Read the model definition and answer for the solid it produces. Units are mm, in the model's axes. A direction names the side the tool comes from. Give positions to 0.01 mm unless a question says otherwise; leave off trailing zeros. Write each loop counter-clockwise with the first axis right and the second up, starting at its lowest first coordinate (ties: lowest second). Pieces come first, ordered by that corner, then holes. Notation, with made-up numbers: (-29.5, -23) - (24.5, -23) arc R24 ccw to (24.5, 12) - close; hole circle Ø5 at (29, 60). An arc over 180 degrees is marked (long way). Answer as CSV lines item,"result".
```python
from build123d import *

# Parameters (mm, degrees)
F1_DEPTH      = 9
F1_DEPTH_BACK = 9
F3_DEPTH      = 25
F3_DEPTH_BACK = 25
F5_DEPTH      = 25
F5_DEPTH_BACK = 25
F6_R          = 2.5
F7_DEPTH      = 25
F7_DEPTH_BACK = 25


with BuildPart() as f1:
    # F0 (on Top) → F1 (new body, two sides)
    with BuildSketch(Plane.XY) as f1_sk:
        with BuildLine():
            ThreePointArc((-0.5590957934, 20), (-0.139801245, 10.0039065883), (0, 0))
            ThreePointArc((0, 0), (-0.139801245, -10.0039065883), (-0.5590957934, -20))
            Line((-0.5590957934, -20), (39, -20))
            Line((39, -20), (39, 20))
            Line((39, 20), (-0.5590957934, 20))
        make_face()
    extrude(amount=F1_DEPTH)
    extrude(f1_sk.sketch, amount=-F1_DEPTH_BACK)

    # F2 (on Front) → F3 (cut, two sides)
    with BuildSketch(Plane.XZ) as f3_sk:
        with BuildLine():
            Line((-2.6374068111, -9), (24, -9))
            Line((24, -9), (17.9378221735, 1.5))
            ThreePointArc((17.9378221735, 1.5), (16.1076951546, 3.3301270189), (13.6076951546, 4))
            Line((13.6076951546, 4), (-2.6374068111, 4))
            Line((-2.6374068111, 4), (-2.6374068111, -9))
        make_face()
    extrude(amount=-F3_DEPTH, mode=Mode.SUBTRACT)
    extrude(f3_sk.sketch, amount=F3_DEPTH_BACK, mode=Mode.SUBTRACT)

    # F4 (on Top) → F5 (cut, two sides)
    with BuildSketch(Plane.XY) as f5_sk:
        with BuildLine():
            ThreePointArc((19, -5), (20.4644660941, -8.5355339059), (24, -10))
            Line((24, -10), (41.5962561965, -10))
            Line((41.5962561965, -10), (41.5962561965, 10))
            Line((41.5962561965, 10), (24, 10))
            ThreePointArc((24, 10), (20.4644660941, 8.5355339059), (19, 5))
            Line((19, 5), (19, 0))
            Line((19, 0), (19, -5))
        make_face()
    extrude(amount=-F5_DEPTH, mode=Mode.SUBTRACT)
    extrude(f5_sk.sketch, amount=F5_DEPTH_BACK, mode=Mode.SUBTRACT)

    # F6 (on Front) → F7 (cut, two sides)
    with BuildSketch(Plane.XZ) as f7_sk:
        with Locations((32, -5)):
            Circle(F6_R)
    extrude(amount=-F7_DEPTH, mode=Mode.SUBTRACT)
    extrude(f7_sk.sketch, amount=F7_DEPTH_BACK, mode=Mode.SUBTRACT)


solid = f1.part
```
(1) A cutting plane is placed at B-B (x = 28). Write down the section's boundary in (y, z), and give its area (3 significant figures).
Worked out:
outline,"(-20, -9) - (-10, -9) - (-10, 9) - (-20, 9) - close; (10, -9) - (20, -9) - (20, 9) - (10, 9) - close"
area,"360 mm^2"
(2) The mould has two halves that part along X. Classify faces 4 (the flat face through (31, 15, -9)), 5 (the flat face through (18.32, -0.28, 0.84)), 6 (the cylindrical face through (31.67, -14.93, -2.52)): +X half, -X half, draft (parallel to the pull), parting line (faces both ways), or undercut.
Worked out:
face 4,"draft"
face 5,"-X half"
face 6,"undercut"
(3) A cutting plane is placed at C-C (z = -3.25). Write down the section's boundary in (x, y).
Worked out:
outline,"(20.68, -20) - (30.21, -20) - (30.21, -10) - (24, -10) arc R5 cw to (20.68, -8.74) - close; (20.68, 8.74) arc R5 cw to (24, 10) - (30.21, 10) - (30.21, 20) - (20.68, 20) - close; (33.79, -20) - (39, -20) - (39, -10) - (33.79, -10) - close; (33.79, 10) - (39, 10) - (39, 20) - (33.79, 20) - close"
(4) For faces 1 (the flat face through (7, 0, 4)), 2 (the cylindrical face through (21, -9, 2)), 3 (the flat face through (39, 15, 0)), determine the directions among +Z, -Z, +X, -X, +Y, -Y from which every point of the face is accessible in a straight line to the end or side of a thin tool.
Worked out:
face 1,"-Z, -X, +Y, -Y"
face 2,"+Z, -Z, +X"
face 3,"+Z, -Z, +X, +Y, -Y"
(5) Find the intervals of material crossed by L1, parallel to Z at x = 32, y = -16; L2, parallel to Y at x = 29.5, z = 1; L3, parallel to X at y = -12.75, z = -5, in increasing order.
Worked out:
L1,"z = -9 to -7.5, -2.5 to 9"
L2,"y = -20 to -10, 10 to 20"
L3,"x = 21.69 to 29.5, 34.5 to 39"
(6) A cutting plane is placed at D-D (y = 17.5). Write down the section's boundary in (x, z), and give its area (3 significant figures).
Worked out:
outline,"(-0.43, 4) - (13.61, 4) arc R5 cw to (17.94, 1.5) - (24, -9) - (39, -9) - (39, 9) - (-0.43, 9) - close; hole circle Ø5 at (32, -5)"
area,"423 mm^2"
(7) A cutting plane is placed at A-A (x = 32). Write down the section's boundary in (y, z), and give its area (3 significant figures).
Worked out:
outline,"(-20, -9) - (-10, -9) - (-10, -7.5) - (-20, -7.5) - close; (-20, -2.5) - (-10, -2.5) - (-10, 9) - (-20, 9) - close; (10, -9) - (20, -9) - (20, -7.5) - (10, -7.5) - close; (10, -2.5) - (20, -2.5) - (20, 9) - (10, 9) - close"
area,"260 mm^2"
(8) Each of these flat-tipped pins is pushed along its axis until it touches: P1, Ø3, axis at x = 4, y = -5, coming from the -Z side; P2, Ø15.5, axis at x = 8.5, y = 7.5, coming from the -Z side; P3, Ø4, axis at x = 32, z = -5, coming from the -Y side; P4, Ø7.5, axis at y = 0.5, z = 2.5, coming from the +X side. Where does it stop, or does it pass through?
Worked out:
P1,"stops at z = 4"
P2,"stops at z = 3.24"
P3,"passes through"
P4,"stops at x = 19"
